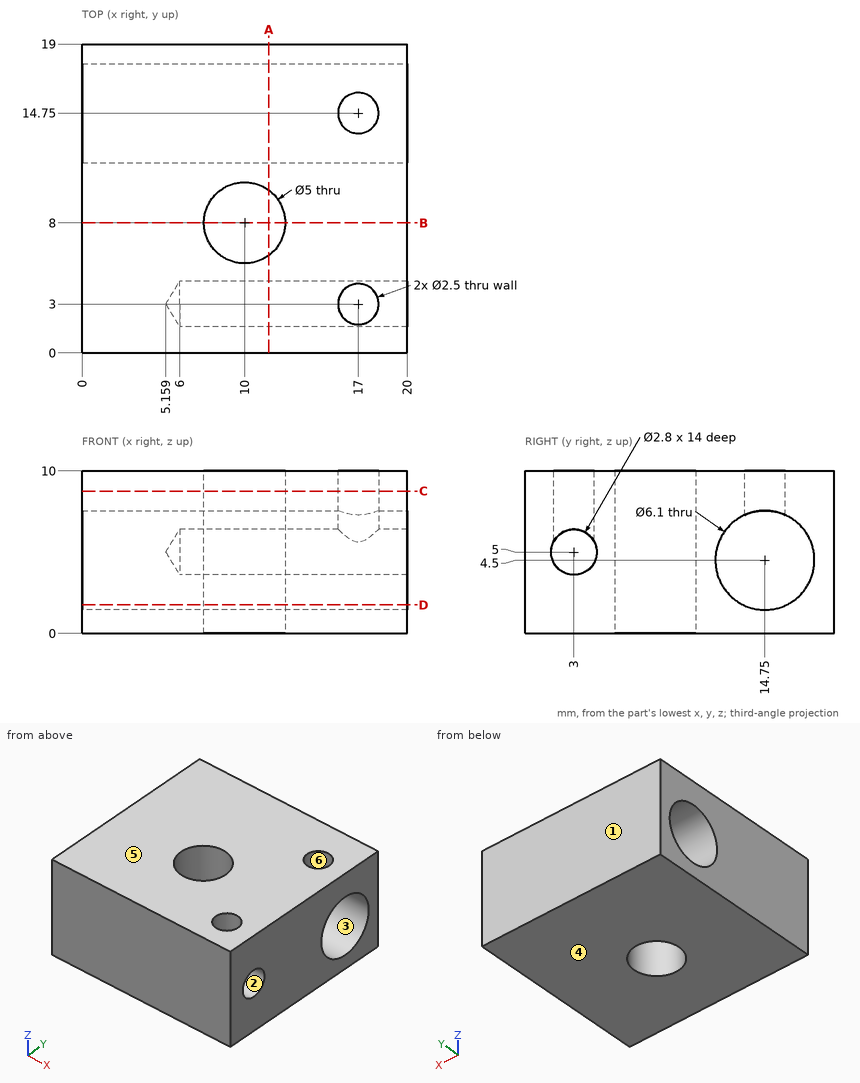
Study the drawing (mm; zero at the part's minimum x, y, z) and answer. A direction names the side the tool comes from. Round coordinates to 2 decimals unless told otherwise and drop trailing zeros. Write each loop counter-clockwise with the first axis right and the second up, starting at its lowest first coordinate (ties: lowest second). Pieces come first, ordered by that corner, then holes. Notation, with made-up numbers: (71, 5.5) - (95, 5.5) arc R16 ccw to (95, 36.5) - close; hole circle Ø4 at (-13.5, 87). An arc over 180 degrees is marked (long way). Return JSON: item names as keys, results as strings. Group by question number.
Q1. The mould has two halves that part along Y. Classify the marked faces 1, 2, 3 and 4: released by +Y, released by -Y, zero draft, split by the parting line, or undercut.
Q2. For the marked faces 5 and 6, determine the directions among +Z, -Z, +X, -X, +Y, -Y from which every point of the face is accessible in a straight line to the end or side of a thin tool.
Q3. Find the intervals of material crossed by L1, parallel to Y at x = 17, z = 9.05; L2, parallel to Z at x = 5.5, y = 14.75; L3, parallel to Y at x = 15, z = 5, in increasing order.
Q4. This flat-tipped pin is pushed along its axis until it touches: pin 1 Ø3.5 at (y, z) = (14.75, 4.5) entering from +X. Where does it stop, or does it pass through?
Q5. The part is cut by section D-D on z = 1.75. Write down the section's boundary in (x, y), then the cut area to 3 significant figures.
Q6. The part is cut by section C-C on z = 8.75. Write down the section's boundary in (x, y), then the cut area to 3 significant figures.
Q7. The part is cut by section A-A on x = 11.5. Write down the section's boundary in (y, z), then the cut area to 3 significant figures.
Q8. The part is cut by section B-B on y = 8. Write down the section's boundary in (x, z), then the cut area to 3 significant figures.
Solved:
{
 "1": {"face 1": "released by +Y", "face 2": "undercut", "face 3": "undercut", "face 4": "zero draft"},
 "2": {"face 5": "+Z, +X, -X, +Y, -Y", "face 6": "+Z"},
 "3": {"L1": "0 to 1.75, 4.25 to 13.5, 16 to 19", "L2": "0 to 1.45, 7.55 to 10", "L3": "0 to 1.6, 4.4 to 11.74, 17.76 to 19"},
 "4": {"pin 1": "through"},
 "5": {"outline": "(0, 0) - (20, 0) - (20, 13.43) - (0, 13.43) - close; (0, 16.07) - (20, 16.07) - (20, 19) - (0, 19) - close; hole circle Ø5 at (10, 8)", "area": "308 mm²"},
 "6": {"outline": "(0, 0) - (20, 0) - (20, 19) - (0, 19) - close; hole circle Ø5 at (10, 8); hole circle Ø2.5 at (17, 3); hole circle Ø2.5 at (17, 14.75)", "area": "351 mm²"},
 "7": {"outline": "(0, 0) - (6, 0) - (6, 10) - (0, 10) - close; (10, 0) - (19, 0) - (19, 10) - (10, 10) - close; hole circle Ø2.8 at (3, 5); hole circle Ø6.1 at (14.75, 4.5)", "area": "115 mm²"},
 "8": {"outline": "(0, 0) - (7.5, 0) - (7.5, 10) - (0, 10) - close; (12.5, 0) - (20, 0) - (20, 10) - (12.5, 10) - close", "area": "150 mm²"}
}
